```python
from build123d import *

# Parameters (mm, degrees)
F0_W     = 740
F0_H     = 301.15
F1_DEPTH = 5
F0_W_2   = 750
F0_H_2   = 311.15
F2_DEPTH = 312.5
F3_R     = 5


with BuildPart() as f1:
    # F0 (on Top) → F1 (new body)
    with BuildSketch(Plane.XY):
        with Locations((375, 155.575)):
            Rectangle(F0_W, F0_H)
    extrude(amount=F1_DEPTH)

    # F0 (on Top) → F2 (join)
    with BuildSketch(Plane.XY):
        with Locations((375, 155.575)):
            Rectangle(F0_W_2, F0_H_2)
        with Locations((375, 155.575)):
            Rectangle(F0_W, F0_H, mode=Mode.SUBTRACT)
    extrude(amount=F2_DEPTH)

    # F3
    f3_edges = [f1.edges().sort_by_distance(p)[0] for p in [
        (375, 306.15, 5),
        (5, 155.575, 5),
        (375, 5, 5),
        (745, 155.575, 5),
        (5, 306.15, 158.75),
        (5, 5, 158.75),
        (745, 306.15, 158.75),
        (745, 5, 158.75),
    ]]
    fillet(f3_edges, radius=F3_R)


solid = f1.part
```
Could you check a few things on this model? Use its own coordinates, in mm. A direction names the side the tool comes from. Give positions to 0.01 mm unless a question says otherwise; leave off trailing zeros. Loops run counter-clockwise (first coordinate to the right, second up) from the corner with the lowest first, then second, coordinate; pieces in that order, holes last. Notation, with made-up numbers: (-26, 16.5) - (-11, 16.5) arc R27 cw to (-11, 32.5) - close; hole circle Ø6 at (14.5, 18.5). An arc over 180 degrees is marked (long way). Answer in a Markdown table with one row per item. Add a question column.
Q1. Which directions (+Z, -Z, +X, -X, +Y, -Y) give clear straight access to the entire face, cutting with the end or side of a thin tool? Please do faces 1 (the face through (370, 306.15, 159)), 2 (the face through (370, 158, 0)).
Q2. If we section it at B-B (y = 47): List the corners of the cut face in (x, z) for me.
Q3. If we section it at A-A (z = 244): List the corners of the cut face in (x, y) for me.
Q4. For pin 1 (4 mm diameter, centred on x = 163.5, y = 208.5, fed in from +Z), with a flat end and sliding along its axis, tell me the tip position at first contact or that it passes through.
Q5. If we section it at C-C (x = 702.5): List the corners of the cut face in (y, z) for me, plus the area to 3 significant figures.
Q6. Please list where these lines run through material, in increasing order: L1, parallel to X at y = 76.5, z = 232; L2, parallel to Y at x = 193, z = 126.5; L3, parallel to Z at x = 150, y = 263.5. Write a range as from..to.
Q7. We'd pull the mould along X, two halves only. Please class faces 3 (the face through (370, 5, 159)), 4 (the face through (370, 0, 154)), 5 (the face through (750, 153, 154)): +X half, -X half, draft (parallel to the pull), parting line (faces both ways), or undercut.
The answers:
| question | item | result |
|---|---|---|
| 1 | face 1 | +Z |
| 1 | face 2 | -Z, +X, -X, +Y, -Y |
| 2 | outline | (0, 0) - (750, 0) - (750, 312.5) - (745, 312.5) - (745, 10) arc R5 cw to (740, 5) - (10, 5) arc R5 cw to (5, 10) - (5, 312.5) - (0, 312.5) - close |
| 3 | outline | (0, 0) - (750, 0) - (750, 311.15) - (0, 311.15) - close; hole (5, 10) arc R5 ccw to (10, 5) - (740, 5) arc R5 ccw to (745, 10) - (745, 301.15) arc R5 ccw to (740, 306.15) - (10, 306.15) arc R5 ccw to (5, 301.15) - close |
| 4 | pin 1 | stops at z = 5 |
| 5 | outline | (0, 0) - (311.15, 0) - (311.15, 312.5) - (306.15, 312.5) - (306.15, 10) arc R5 cw to (301.15, 5) - (10, 5) arc R5 cw to (5, 10) - (5, 312.5) - (0, 312.5) - close |
| 5 | area | 4,640 mm^2 |
| 6 | L1 | x = 0..5, 745..750 |
| 6 | L2 | y = 0..5, 306.15..311.15 |
| 6 | L3 | z = 0..5 |
| 7 | face 3 | undercut |
| 7 | face 4 | draft |
| 7 | face 5 | +X half |
